from build123d import *

# Parameters (mm, degrees)
SKETCH_1_W               = 42
SKETCH_1_H               = 42
EXTRUDE_1_DEPTH          = 17
CUT_EXTRUDE_1_DEPTH      = 8
PATTERN_CIRCULAR_1_COUNT = 4
FILLET_1_R               = 16
CHAMFER_1_SIZE           = 5
SKETCH_3_R               = 11
EXTRUDE_2_DEPTH          = 2
EXTRUDE_3_DEPTH          = 8.2


with BuildPart() as part:
    # 스케치1 → 보스-돌출1 (new, symmetric)
    with BuildSketch(Plane(origin=(0, 0, 0), x_dir=(1, 0, 0), z_dir=(0, 1, 0))):
        Rectangle(SKETCH_1_W, SKETCH_1_H)
    extrude(amount=EXTRUDE_1_DEPTH, both=True)

    # 스케치2 → 컷-돌출1 (cut, symmetric)
    with BuildSketch(Plane(origin=(0, 0, 0), x_dir=(1, 0, 0), z_dir=(0, 1, 0))):
        Polygon((-21, 13), (-13, 21), (-21, 21), align=None)
    cut_extrude_1 = extrude(amount=CUT_EXTRUDE_1_DEPTH, both=True, mode=Mode.SUBTRACT)

    # 원형 패턴1: 컷-돌출1 ×4 about axis
    pattern_circular_1_axis = Axis((0, 0, 0), (0, 1, 0))
    for i in range(1, PATTERN_CIRCULAR_1_COUNT):
        add(cut_extrude_1.rotate(pattern_circular_1_axis, i * 360 / PATTERN_CIRCULAR_1_COUNT), mode=Mode.SUBTRACT)

    # 필렛1
    # the kernel refuses this fillet: 16 mm, written as the material it takes off along each edge
    with BuildSketch(Plane(origin=(21, -8, -13), x_dir=(0, 0, 1), z_dir=(0, 1, 0)), Plane(origin=(13, 8, -21), x_dir=(-1, 0, 0), z_dir=(0, -1, 0)), Plane(origin=(-21, 8, -13), x_dir=(0, 0, 1), z_dir=(0, -1, 0)), Plane(origin=(-13, 8, 21), x_dir=(1, 0, 0), z_dir=(0, -1, 0)), Plane(origin=(13, -8, 21), x_dir=(-1, 0, 0), z_dir=(0, 1, 0)), Plane(origin=(21, 8, 13), x_dir=(0, 0, -1), z_dir=(0, -1, 0))) as fillet_1_piece_1:
        with BuildLine():
            CenterArc((FILLET_1_R * 0.414213562373, -FILLET_1_R), FILLET_1_R, 90, 45)
            Line((-FILLET_1_R * 0.292893218813, -FILLET_1_R * 0.292893218813), (0, 0))
            Line((0, 0), (FILLET_1_R * 0.414213562373, 0))
        make_face()
    extrude(amount=16, mode=Mode.SUBTRACT)
    with BuildSketch(Plane(origin=(-13, -8, -21), x_dir=(-0.7071067811865475, 0, 0.7071067811865477), z_dir=(0, 1, 0)), Plane(origin=(-21, -8, 13), x_dir=(0.7071067811865472, 0, 0.7071067811865478), z_dir=(0, 1, 0))) as fillet_1_piece_2:
        with BuildLine():
            CenterArc((FILLET_1_R * 0.414213562373, FILLET_1_R), FILLET_1_R, 225, 45)
            Line((-FILLET_1_R * 0.292893218813, FILLET_1_R * 0.292893218813), (0, 0))
            Line((0, 0), (FILLET_1_R * 0.414213562373, 0))
        make_face()
    extrude(amount=16, mode=Mode.SUBTRACT)

    # 모따기1
    chamfer_1_edges = [part.edges().sort_by_distance(p)[0] for p in [
        (-21, -12.5, -21),
        (21, -12.5, 21),
        (-21, -12.5, 21),
        (21, -12.5, -21),
        (21, 12.5, 21),
        (-21, 12.5, 21),
        (-21, 12.5, -21),
        (21, 12.5, -21),
    ]]
    chamfer(chamfer_1_edges, length=CHAMFER_1_SIZE)

    # 스케치3 → 보스-돌출2 (add)
    with BuildSketch(Plane(origin=(0, 17, 0), x_dir=(1, 0, 0), z_dir=(0, 1, 0))):
        with Locations(Location((0, 0, 0), (0, 0, 270))):
            Circle(SKETCH_3_R)
    extrude(amount=EXTRUDE_2_DEPTH)

    # 스케치4 → 보스-돌출3 (add)
    with BuildSketch(Plane(origin=(0, 19, 0), x_dir=(1, 0, 0), z_dir=(0, 1, 0))):
        with BuildLine():
            Line((0, 2), (-1.5, 2))
            ThreePointArc((-1.5, 2), (-2.371708245, -0.790569415), (0, -2.5))
            Line((0, -2.5), (0, 2))
        make_face()
        with BuildLine():
            Line((1.5, 2), (0, 2))
            Line((0, 2), (0, -2.5))
            ThreePointArc((0, -2.5), (1.767766953, -1.767766953), (2.5, 0))
            ThreePointArc((2.5, 0), (2.236067977, 1.118033989), (1.5, 2))
        make_face()
    extrude(amount=EXTRUDE_3_DEPTH)


solid = part.part
Design review of the part built by this model. Coordinates are the model's own, in mm. A direction names the side the tool comes from. Coordinates: 2 decimals unless noted, no trailing zeros. Loops run counter-clockwise (first coordinate to the right, second up) from the corner with the lowest first, then second, coordinate; pieces in that order, holes last.
Item 1: Add section B-B (z = 1.5). Write out the cut boundary in (x, y), and give its area (3 significant figures).
Completed:
outline: (-21, -17) - (21, -17) - (21, 17) - (10.9, 17) - (10.9, 19) - (2, 19) - (2, 27.2) - (-2, 27.2) - (-2, 19) - (-10.9, 19) - (-10.9, 17) - (-21, 17) - close
area: 1,500 mm2
Item 2: Clearance check with flat-ended pins moving along their axes: pin 1 (5 mm diameter, centred on y = -1, z = 15.5, fed in from -X); pin 2 (16 mm diameter, centred on x = 13, z = 13, fed in from +Y); pin 3 (11.5 mm diameter, centred on x = 10.5, z = -15.5, fed in from +Y). State where each tip first meets the part, or that it passes through.
Completed:
pin 1: stops at x = -19.56
pin 2: stops at y = 19
pin 3: stops at y = 17
Item 3: Draft analysis for pull direction Y (two halves, no side actions). For faces 1 (the flat face through (-18, 12, 19)), 2 (the flat face through (0, -17, 0)), 3 (the cylindrical face through (11.97, 0.11, -19.99)), state which applies: pulls with the +Y half, pulls with the -Y half, needs draft (parallel to the pull), parting line crosses it, or undercut.
Completed:
face 1: needs draft
face 2: pulls with the -Y half
face 3: undercut
Item 4: Add section C-C (x = 10). Write out the cut boundary in (y, z).
Completed:
outline: (-17, -21) - (-8, -21) - (-8, -20.58) - (8, -20.58) - (8, -21) - (17, -21) - (17, -4.58) - (19, -4.58) - (19, 4.58) - (17, 4.58) - (17, 21) - (8, 21) - (8, 20.58) - (-8, 20.58) - (-8, 21) - (-17, 21) - close
Item 5: Add section D-D (y = 23). Write out the cut boundary in (x, z).
Completed:
outline: (-1.5, -2) - (1.5, -2) arc R2.5 ccw (long way) to start
Item 6: For faces 4 (the cylindrical face through (-19.99, -0.11, 11.97)), 5 (the cylindrical face through (19.99, 0.11, 11.97)), 6 (the flat face through (17, -8, -18)), 7 (the cylindrical face through (-11.97, -0.11, -19.99)), list the 3-axis set-ups (+Z, -Z, +X, -X, +Y, -Y) from which the entire face can be reached by the end or side of a thin tool; tool diameter is ignored.
Completed:
face 4: +Z, -X
face 5: +Z, +X
face 6: -Z, +X
face 7: -Z, -X
Item 7: Wall thickness on L1, parallel to Y at x = 19.5, z = -14.5; L2, parallel to Y at x = -0.5, z = 7; L3, parallel to Y at x = 18, z = 6: over which ranges is each line inside the solid? List them lowest first.
Completed:
L1: y = -17 to -8, 8 to 17
L2: y = -17 to 19
L3: y = -17 to 17
Item 8: Add section A-A (y = 12). Write out the cut boundary in (x, z).
Completed:
outline: (-21, -16) - (-16, -21) - (16, -21) - (21, -16) - (21, 16) - (16, 21) - (-16, 21) - (-21, 16) - close
